The listing builds one solid part. Answer for the finished solid, in the listing's coordinates (mm). A direction names the side the tool comes from. Round coordinates to 2 decimals unless told otherwise and drop trailing zeros. Order: outer loops, then holes, each group sorted by start corner. A loop starts at its lowest first (then second) coordinate and runs counter-clockwise, first axis right, second up. Notation, with made-up numbers: (78, 44.25) -> (88, 44.25) arc R14 ccw to (88, 70.25) -> close; hole circle Ø9 at (-15, 10). An arc over 180 degrees is marked (long way). Return JSON: item names as keys, results as strings. Group by question number.
(1) Consider line 1 (X direction, y = -16.1, z = 3); line 2 (Z direction, x = 6.5, y = 4.5); line 3 (Z direction, x = -10, y = 1). Determine where each line is inside the solid, lowest interval first. Write a range as [from, to].
(2) Which of the six approach directions +Z, -Z, +X, -X, +Y, -Y give full straight-line access (tool end or side, diameter ignored) to faces 4 (the face through (17, -17, 6)), 5 (the face through (4.38, -8.43, 2.93)), 6 (the face through (-17, -17, 6))?
(3) The part is cut by section A-A (z = 33). Determine the outline of the cut face in (x, y), plus the area to 3 significant figures.
(4) The part is cut by section C-C (y = -1.5). Determine the outline of the cut face in (x, z).
(5) Determine the mould class of faces 1 (the face through (-23, -18, 3)), 2 (the face through (1.802, 5.723, 29.036)), 3 (the face through (17, -17, 30)) for opening direction X: +X half, -X half, draft (parallel to the pull), parting line (faces both ways), or undercut.
(6) The part is cut by section B-B (x = 0). Determine the outline of the cut face in (y, z).
(7) Each of these flat-tipped pins is pushed along its axis until it touches: pin 1 (1 mm diameter, centred on x = 3.5, y = 5, fed in from +Z); pin 2 (16 mm diameter, centred on x = -2, z = 18, fed in from +Y); pin 3 (2 mm diameter, centred on x = 12.5, z = 11.5, fed in from +Y). Where does it stop, or does it pass through?
(8) The part is cut by section D-D (z = 27). Determine the outline of the cut face in (x, y), plus the area to 3 significant figures.
from build123d import *

# Parameters (mm, degrees)
CROQUIS1_R              = 9.5
SALIENTE_EXTRUIR1_DEPTH = 36
CROQUIS2_W              = 20.1
CROQUIS2_H              = 28
CORTAR_EXTRUIR2_DEPTH   = 49.703182648
CROQUIS3_R              = 9.5
CROQUIS3_R_2            = 6
SALIENTE_EXTRUIR2_DEPTH = 2
SALIENTE_EXTRUIR3_START = -2
CROQUIS4_R              = 9.5
CROQUIS4_R_2            = 6
SALIENTE_EXTRUIR3_DEPTH = 2
SALIENTE_EXTRUIR4_DEPTH = 5
CROQUIS6_R              = 1.5
CORTAR_EXTRUIR3_DEPTH   = 54.981478305
REDONDEO1_R             = 3
REDONDEO2_R             = 3


with BuildPart() as part:
    # Croquis1 → Saliente-Extruir1 (new body)
    with BuildSketch(Plane.XY):
        with BuildLine():
            Line((-13, 0), (-13, -20))
            Line((-13, -20), (13, -20))
            Line((13, -20), (13, 0))
            ThreePointArc((13, 0), (0, 13), (-13, 0))
        make_face()
        Circle(CROQUIS1_R, mode=Mode.SUBTRACT)
    extrude(amount=SALIENTE_EXTRUIR1_DEPTH)

    # Croquis2 → Cortar-Extruir2 (cut, through all)
    with BuildSketch(Plane(origin=(13, 0, 0), x_dir=(0, 0, -1), z_dir=(1, 0, 0))):
        with Locations((-18, -1)):
            Rectangle(CROQUIS2_W, CROQUIS2_H)
    extrude(amount=-CORTAR_EXTRUIR2_DEPTH, mode=Mode.SUBTRACT)

    # Croquis3 → Saliente-Extruir2 (add)
    with BuildSketch(Plane(origin=(0, 0, 28.05), x_dir=(-1, 0, 0), z_dir=(0, 0, -1))):
        with Locations(Location((0, 0, 0), (0, 0, 90))):
            Circle(CROQUIS3_R)
        with Locations(Location((0, 0, 0), (0, 0, 90))):
            Circle(CROQUIS3_R_2, mode=Mode.SUBTRACT)
    extrude(amount=-SALIENTE_EXTRUIR2_DEPTH)

    # Croquis4 → Saliente-Extruir3 (add)
    with BuildSketch(Plane.XY.offset(7.95).offset(SALIENTE_EXTRUIR3_START)):
        Circle(CROQUIS4_R)
        with Locations(Location((0, 0, 0), (0, 0, 90))):
            Circle(CROQUIS4_R_2, mode=Mode.SUBTRACT)
    extrude(amount=SALIENTE_EXTRUIR3_DEPTH)

    # Croquis5 → Saliente-Extruir4 (add)
    with BuildSketch(Plane.XZ.offset(20)):
        with BuildLine():
            Line((13, 36), (20, 36))
            ThreePointArc((20, 36), (23, 33), (20, 30))
            Line((20, 30), (13, 30))
            Line((13, 30), (13, 36))
        make_face()
        with BuildLine():
            Line((13, 0), (20, 0))
            ThreePointArc((20, 0), (23, 3), (20, 6))
            Line((20, 6), (13, 6))
            Line((13, 6), (13, 0))
        make_face()
        with BuildLine():
            Line((-13, 0), (-20, 0))
            ThreePointArc((-20, 0), (-23, 3), (-20, 6))
            Line((-20, 6), (-13, 6))
            Line((-13, 6), (-13, 0))
        make_face()
        with BuildLine():
            Line((-13, 30), (-13, 36))
            Line((-13, 36), (-20, 36))
            ThreePointArc((-20, 36), (-23, 33), (-20, 30))
            Line((-20, 30), (-13, 30))
        make_face()
    extrude(amount=-SALIENTE_EXTRUIR4_DEPTH)

    # Croquis6 → Cortar-Extruir3 (cut, through all)
    with BuildSketch(Plane.XZ.offset(20)):
        with Locations(Location((-20, 33, 0), (0, 0, 270))):
            Circle(CROQUIS6_R)
        with Locations(Location((20, 33, 0), (0, 0, 270))):
            Circle(CROQUIS6_R)
        with Locations(Location((-20, 3, 0), (0, 0, 270))):
            Circle(CROQUIS6_R)
        with Locations(Location((20, 3, 0), (0, 0, 270))):
            Circle(CROQUIS6_R)
    extrude(amount=-CORTAR_EXTRUIR3_DEPTH, mode=Mode.SUBTRACT)

    # Redondeo1
    redondeo1_edges = [part.edges().sort_by_distance(p)[0] for p in [
        (-13, -15, 33),
        (-13, -15, 3),
        (13, -15, 3),
        (13, -15, 33),
    ]]
    fillet(redondeo1_edges, radius=REDONDEO1_R)

    # Redondeo2
    redondeo2_edges = [part.edges().sort_by_distance(p)[0] for p in [
        (-13, -15, 18),
        (13, -15, 18),
    ]]
    fillet(redondeo2_edges, radius=REDONDEO2_R)


solid = part.part
Answer below:
{
 "1": {"line 1": "x = [-23, -21.5], [-18.5, 18.5], [21.5, 23]", "line 2": "z = [5.95, 7.95], [28.05, 30.05]", "line 3": "z = [0, 7.95], [28.05, 36]"},
 "2": {"face 4": "+X, +Y, -Y", "face 5": "-Z", "face 6": "-X, +Y, -Y"},
 "3": {"outline": "(-23, -20) -> (-21.5, -20) -> (-21.5, -15) -> (-23, -15) -> close; (-18.5, -20) -> (18.5, -20) -> (18.5, -15) -> (16, -15) arc R3 cw to (13, -12) -> (13, 0) arc R13 ccw to (-13, 0) -> (-13, -12) arc R3 cw to (-16, -15) -> (-18.5, -15) -> close; (21.5, -20) -> (23, -20) -> (23, -15) -> (21.5, -15) -> close; hole circle Ø19 at (0, 0)", "area": "576 mm²"},
 "4": {"outline": "(-13, 0) -> (-9.38, 0) -> (-9.38, 5.95) -> (-5.81, 5.95) -> (-5.81, 7.95) -> (-13, 7.95) -> close; (-13, 28.05) -> (-5.81, 28.05) -> (-5.81, 30.05) -> (-9.38, 30.05) -> (-9.38, 36) -> (-13, 36) -> close; (5.81, 5.95) -> (9.38, 5.95) -> (9.38, 0) -> (13, 0) -> (13, 7.95) -> (5.81, 7.95) -> close; (5.81, 28.05) -> (13, 28.05) -> (13, 36) -> (9.38, 36) -> (9.38, 30.05) -> (5.81, 30.05) -> close"},
 "5": {"face 1": "-X half", "face 2": "undercut", "face 3": "draft"},
 "6": {"outline": "(-20, 0) -> (-9.5, 0) -> (-9.5, 5.95) -> (-6, 5.95) -> (-6, 7.95) -> (-15, 7.95) -> (-15, 28.05) -> (-6, 28.05) -> (-6, 30.05) -> (-9.5, 30.05) -> (-9.5, 36) -> (-20, 36) -> close; (6, 5.95) -> (9.5, 5.95) -> (9.5, 0) -> (13, 0) -> (13, 7.95) -> (6, 7.95) -> close; (6, 28.05) -> (13, 28.05) -> (13, 36) -> (9.5, 36) -> (9.5, 30.05) -> (6, 30.05) -> close"},
 "7": {"pin 1": "stops at z = 30.05", "pin 2": "stops at y = -15", "pin 3": "stops at y = -15.4"},
 "8": {"outline": "(-13, -20) -> (13, -20) -> (13, -18) arc R3 ccw to (10, -15) -> (-10, -15) arc R3 ccw to (-13, -18) -> close", "area": "126 mm²"}
}
